```python
from build123d import *

# Parameters (mm, degrees)
CROQUIS3_W            = 12.155845656
CROQUIS3_H            = 36.65917603
CORTAR_EXTRUIR1_DEPTH = 21


with BuildPart() as part:
    # Croquis2 → Revolución1 (revolve)
    with BuildSketch(Plane(origin=(0, 0, 0), x_dir=(0, 0, -1), z_dir=(1, 0, 0))):
        with BuildLine():
            Line((0, 0), (-4.7, 0))
            Line((-4.7, 0), (-4.7, 9.902147454))
            ThreePointArc((-4.7, 9.902147454), (-5.319949818, 11.349718348), (-6.795461494, 11.899867931))
            Line((-6.795461494, 11.899867931), (-6.695457392, 11.904646648))
            ThreePointArc((-6.695457392, 11.904646648), (-12.523047033, 14.558265513), (-13.753776425, 20.842197345))
            Line((-13.753776425, 20.842197345), (-12.389960221, 25.555865437))
            ThreePointArc((-12.389960221, 25.555865437), (-11.670480634, 26.598707427), (-10.468759134, 27))
            Line((-10.468759134, 27), (-9.486832981, 27))
            ThreePointArc((-9.486832981, 27), (-9.064255853, 26.767261242), (-9.035079029, 26.285714286))
            ThreePointArc((-9.035079029, 26.285714286), (-8.451542547, 16.654775162), (0, 12))
            Line((0, 12), (0, 0))
        make_face()
    revolve(axis=Axis((0, 22, 0), (0, -1, 0)))

    # Croquis3 → Cortar-Extruir1 (cut)
    with BuildSketch(Plane(origin=(0, 30, 0), x_dir=(1, 0, 0), z_dir=(0, 1, 0))):
        with Locations((-12.077922828, -0.329588015)):
            Rectangle(CROQUIS3_W, CROQUIS3_H)
        with Locations((12.077922828, -0.329588015)):
            Rectangle(CROQUIS3_W, CROQUIS3_H)
    extrude(amount=-CORTAR_EXTRUIR1_DEPTH, mode=Mode.SUBTRACT)


solid = part.part
```
Geometry: final body of the model. Coordinates: model frame, mm. A direction names the side the tool comes from. Coordinates: 2 decimals unless noted, no trailing zeros. Order: outer loops, then holes, each group sorted by start corner. A loop starts at its lowest first (then second) coordinate and runs counter-clockwise, first axis right, second up. Notation, with made-up numbers: (16, -37.5) - (47, -37.5) arc R27 ccw to (47, -0.5) - close; hole circle Ø10 at (74, 76). An arc over 180 degrees is marked (long way). Write each question's results on one line, items separated by ' | '.
1) Section C-C, the plane x = 0. Return loops of the section in (y, z), plus the area to 3 significant figures.
Results list:
outline: (0, -4.7) - (9.9, -4.7) arc R2 cw to (11.9, -6.8) - (11.9, -6.7) arc R7 ccw to (20.84, -13.75) - (25.56, -12.39) arc R2 ccw to (27, -10.47) - (27, -9.49) arc R0.5 ccw to (26.29, -9.04) arc R10 cw (long way) to (26.29, 9.04) arc R0.5 ccw to (27, 9.49) - (27, 10.47) arc R2 ccw to (25.56, 12.39) - (20.84, 13.75) arc R7 ccw to (11.9, 6.7) - (11.9, 6.8) arc R2 cw to (9.9, 4.7) - (0, 4.7) - close | area: 248 mm^2
2) Set-up query: faces 1 (the flat face through (0, 0, 0)), 2 (the cylindrical face through (4.59, 5.02, -1.02)). Return all of +Z, -Z, +X, -X, +Y, -Y with unobstructed straight access to the full face (end or side cutting, diameter ignored); none if empty.
Results list:
face 1: +Z, -Z, +X, -X, -Y | face 2: -Y
3) Section A-A, the plane y = 17. Return loops of the section in (x, z) (1 decimal), plus the area to 3 significant figures.
Results list:
outline: (-6, -12.4) arc R13.8 ccw to (6, -12.4) - (6, -6.2) arc R8.7 cw to (-6, -6.2) - close; (-6, 6.2) arc R8.7 cw to (6, 6.2) - (6, 12.4) arc R13.8 ccw to (-6, 12.4) - close | area: 130 mm^2
4) Section B-B, the plane z = 0. Return loops of the section in (x, y).
Results list:
outline: (-6, 11.78) arc R2 cw to (-4.7, 9.9) - (-4.7, 0) - (4.7, 0) - (4.7, 9.9) arc R2 cw to (6, 11.78) - (6, 14) arc R10 cw to (-6, 14) - close
5) Line query: line 1 (Z direction, x = -1.5, y = 13.75); line 2 (X direction, y = 13.75, z = 2); line 3 (Z direction, x = 4.75, y = 17.25). Output: solid intervals per line, ascending. Write a range as from..to.
Results list:
line 1: -11.68..-5.45, 5.45..11.68 | line 2: -6..-5.29, 5.29..6 | line 3: -12.99..-7.41, 7.41..12.99
6) Pin query (flat end, axial travel): pin 1 (5 mm diameter, centred on x = -2, y = 5.5, fed in from +Z); pin 2 (1 mm diameter, centred on x = -0.5, z = 11, fed in from -Y); pin 3 (8 mm diameter, centred on y = 10.5, z = -9.5, fed in from +X); pin 4 (4 mm diameter, centred on x = 0.5, z = -1, fed in from +Y). Return the tip coordinate at first contact, or that it passes through.
Results list:
pin 1: z = 4.7 | pin 2: y = 12.82 | pin 3: x = 6 | pin 4: y = 12.5
7) Section D-D, the plane y = 22.5. Return loops of the section in (x, z), plus the area to 3 significant figures.
Results list:
outline: (-6, -11.84) arc R13.27 ccw to (6, -11.84) - (6, -7.98) arc R9.99 cw to (-6, -7.98) - close; (-6, 7.98) arc R9.99 cw to (6, 7.98) - (6, 11.84) arc R13.27 ccw to (-6, 11.84) - close | area: 83.0 mm^2
